Part model, mm, in its own coordinate system. Face numbers are marked on the shaded views. A direction names the side the tool comes from. Round coordinates to 2 decimals unless told otherwise and drop trailing zeros. Order: outer loops, then holes, each group sorted by start corner. A loop starts at its lowest first (then second) coordinate and runs counter-clockwise, first axis right, second up. Notation, with made-up numbers: (43, 69.5) - (63, 69.5) arc R26 ccw to (63, 101.5) - close; hole circle Ø5 at (47, 45). An arc over 180 degrees is marked (long way). Answer as a JSON object with one key per item and string values.
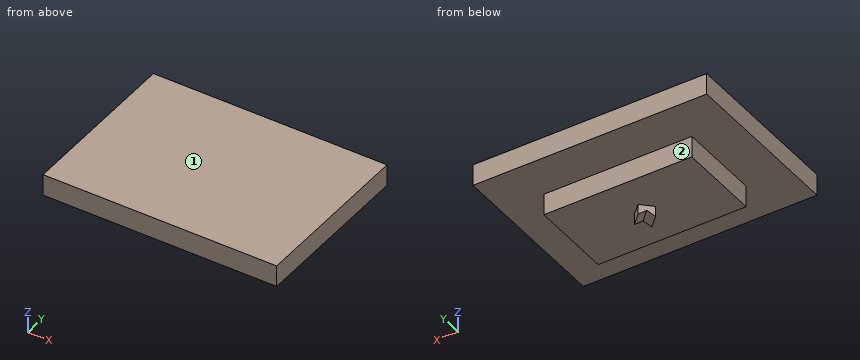
```python
from build123d import *

# Parameters (mm, degrees)
SKIZZE1_W                       = 6.912
SKIZZE1_H                       = 3.888
AUFSATZ_LINEAR_AUSTRAGEN1_DEPTH = 1
SKIZZE2_W                       = 10.912
SKIZZE2_H                       = 7.888
AUFSATZ_LINEAR_AUSTRAGEN2_DEPTH = 1
AUFSATZ_LINEAR_AUSTRAGEN3_DEPTH = 0.48
SCHNITT_LINEAR_AUSTRAGEN1_DEPTH = 40.48


with BuildPart() as part:
    # Skizze1 → Aufsatz-Linear austragen1 (new body)
    with BuildSketch(Plane.XY):
        with Locations((3.456, 1.944)):
            Rectangle(SKIZZE1_W, SKIZZE1_H)
    extrude(amount=AUFSATZ_LINEAR_AUSTRAGEN1_DEPTH)

    # Skizze2 → Aufsatz-Linear austragen2 (add)
    with BuildSketch(Plane.XY.offset(1)):
        with Locations((3.456, 1.944)):
            Rectangle(SKIZZE2_W, SKIZZE2_H)
    extrude(amount=AUFSATZ_LINEAR_AUSTRAGEN2_DEPTH)

    # Skizze3 → Aufsatz-Linear austragen3 (add)
    with BuildSketch(Plane(origin=(0, 0, 0), x_dir=(-1, 0, 0), z_dir=(0, 0, -1))):
        Polygon((-3.956, 1.944), (-3.456, 2.444), (-2.961061255, 1.949061255), (-3.461061255, 1.449061255), align=None)
    extrude(amount=AUFSATZ_LINEAR_AUSTRAGEN3_DEPTH)

    # Skizze6 → Schnitt-Linear austragen1 (cut)
    with BuildSketch(Plane(origin=(1.006, -1.006, 0), x_dir=(0, 0, -1), z_dir=(0.7071067811865474, -0.7071067811865477, 0))):
        Polygon((0.48, 4.171930009), (0.24, 3.821955466), (0.48, 3.471980924), align=None)
    extrude(amount=-SCHNITT_LINEAR_AUSTRAGEN1_DEPTH, mode=Mode.SUBTRACT)


solid = part.part
```
Item 1: Probe L1, parallel to Y at x = 2, z = 0.65; L2, parallel to Z at x = 6, y = 4.75; L3, parallel to Z at x = 0.5, y = 0.75. List the from-to ranges inside material, lowest first. Write a range as from..to.
Taken from the geometry:
{"L1": "0..3.89", "L2": "1..2", "L3": "0..2"}
Item 2: Cut at B-B (y = 3.75). Write the cut outline in (x, z), plus the area to 3 significant figures.
Taken from the geometry:
{"outline": "(-2, 1) - (0, 1) - (0, 0) - (6.91, 0) - (6.91, 1) - (8.91, 1) - (8.91, 2) - (-2, 2) - close", "area": "17.8 mm2"}
Item 3: Cut at A-A (x = 6.25). Write the cut outline in (y, z).
Taken from the geometry:
{"outline": "(-2, 1) - (0, 1) - (0, 0) - (3.89, 0) - (3.89, 1) - (5.89, 1) - (5.89, 2) - (-2, 2) - close"}
Item 4: Tool access for the marked faces 1 and 2: list every direction of +Z, -Z, +X, -X, +Y, -Y with a clear straight run to the whole face (end or side of a thin tool).
Taken from the geometry:
{"face 1": "+Z, +X, -X, +Y, -Y", "face 2": "-Z, +X, -X, +Y"}
Item 5: Cut at C-C (z = 0.2). Write the cut outline in (x, y), plus the area to 3 significant figures.
Taken from the geometry:
{"outline": "(0, 0) - (6.91, 0) - (6.91, 3.89) - (0, 3.89) - close", "area": "26.9 mm2"}
Item 6: Cut at D-D (x = -1). Write the cut outline in (y, z).
Taken from the geometry:
{"outline": "(-2, 1) - (5.89, 1) - (5.89, 2) - (-2, 2) - close"}
Item 7: Drop flat-ended pins along their axis: P1, Ø0.8, axis at x = 3.5, z = 0.5, coming from the -Y side; P2, Ø1.2, axis at x = 4.5, y = 2, coming from the -Z side; P3, Ø0.5, axis at y = 1, z = 0.5, coming from the -X side; P4, Ø0.8, axis at y = 2.5, z = 0.5, coming from the +X side. Give the stop position or say it passes through.
Taken from the geometry:
{"P1": "y = 0", "P2": "z = -0.48", "P3": "x = 0", "P4": "x = 6.91"}
